Here's how the part is built. I have some questions about the finished solid (model axes, mm). A direction names the side the tool comes from. Give positions to 0.01 mm unless a question says otherwise; leave off trailing zeros. Loops run counter-clockwise (first coordinate to the right, second up) from the corner with the lowest first, then second, coordinate; pieces in that order, holes last.
Q1. Thinking about a two-plate mould opening in Z: for faces 1 (the face through (-68, 52, 0)), 2 (the face through (-67.56, 32.18, 8.35)), 3 (the face through (-68, 52, 44)), 4 (the face through (-75, 54.741, 22)), which applies, pulls with the +Z half, pulls with the -Z half, needs draft (parallel to the pull), parting line crosses it, or undercut?
Q2. Suppose I cut it at A-A (z = 8). List the corners of the cut face in (x, y) for me, and give its area (3 significant figures).
Q3. Suppose I cut it at C-C (z = 18). List the corners of the cut face in (x, y) for me.
Q4. Suppose I cut it at B-B (y = 56). List the corners of the cut face in (x, z) for me.
Q5. Suppose I cut it at D-D (x = -77.5). List the corners of the cut face in (y, z) for me.
Q6. I'm going to push flat-ended pins straight in: P1, Ø3.5, axis at x = -73.09, z = 15.57, coming from the +Y side; P2, Ø5, axis at x = -73.09, z = 27.57, coming from the -Y side; P3, Ø3.5, axis at y = 33.74, z = 40, coming from the -X side. Where does each tip first touch, or does it pass through?
Q7. I need wall thicknesses on probe 1 along Y at (x, z) = (-67.15, 40); probe 2 along Z at (x, y) = (-71.75, 57.5); probe 3 along Y at (x, z) = (-78.5, 36.5). Which ranges of each line are inside material? Lowest first, please.
Q8. For faces 5 (the face through (-67.6, 32.3, 39.3)), 6 (the face through (-69.585, 41, 22)), which set-ups out of +Z, -Z, +X, -X, +Y, -Y let a thin tool reach every point of the face, with its end or its side?
```python
from build123d import *

# Parameters (mm, degrees)
BOSS_EXTRUDE1_DEPTH = 44
SKETCH3_R           = 1.6
CUT_EXTRUDE2_DEPTH  = 10
SKETCH2_R           = 1.6
CUT_EXTRUDE3_DEPTH  = 10


with BuildPart() as part:
    # Sketch1 → Boss-Extrude1 (new body)
    with BuildSketch(Plane.XY):
        Polygon((-80.585156419, 60.740798274), (-80.585156419, 54.740798274), (-69.585156419, 54.740798274), (-69.585156419, 26.740798274), (-65.585156419, 26.740798274), (-65.585156419, 60.740798274), align=None)
    extrude(amount=BOSS_EXTRUDE1_DEPTH)

    # Sketch3 → Cut-Extrude2 (cut)
    with BuildSketch(Plane(origin=(-65.585156419, 0, 0), x_dir=(0, 0, -1), z_dir=(1, 0, 0))):
        with Locations((-40, 33.740798274)):
            Circle(SKETCH3_R)
        with Locations((-8, 33.740798274)):
            Circle(SKETCH3_R)
    extrude(amount=-CUT_EXTRUDE2_DEPTH, mode=Mode.SUBTRACT)

    # Sketch2 → Cut-Extrude3 (cut)
    with BuildSketch(Plane(origin=(0, 60.740798274, 0), x_dir=(1, 0, 0), z_dir=(0, 1, 0))):
        with Locations(Location((-73.085156419, -3.571673595, 0), (0, 0, 180))):
            Circle(SKETCH2_R)
        with Locations(Location((-73.085156419, -15.571673595, 0), (0, 0, 180))):
            Circle(SKETCH2_R)
        with Locations(Location((-73.085156419, -27.571673595, 0), (0, 0, 180))):
            Circle(SKETCH2_R)
        with Locations(Location((-73.085156419, -39.571673595, 0), (0, 0, 180))):
            Circle(SKETCH2_R)
    extrude(amount=-CUT_EXTRUDE3_DEPTH, mode=Mode.SUBTRACT)


solid = part.part
```
Solutions:
1. face 1: pulls with the -Z half
1. face 2: undercut
1. face 3: pulls with the +Z half
1. face 4: needs draft
2. outline: (-80.59, 54.74) - (-69.59, 54.74) - (-69.59, 35.34) - (-65.59, 35.34) - (-65.59, 60.74) - (-80.59, 60.74) - close; (-69.59, 26.74) - (-65.59, 26.74) - (-65.59, 32.14) - (-69.59, 32.14) - close
2. area: 189 mm2
3. outline: (-80.59, 54.74) - (-69.59, 54.74) - (-69.59, 26.74) - (-65.59, 26.74) - (-65.59, 60.74) - (-80.59, 60.74) - close
4. outline: (-80.59, 0) - (-65.59, 0) - (-65.59, 44) - (-80.59, 44) - close; hole circle Ø3.2 at (-73.09, 3.57); hole circle Ø3.2 at (-73.09, 15.57); hole circle Ø3.2 at (-73.09, 27.57); hole circle Ø3.2 at (-73.09, 39.57)
5. outline: (54.74, 0) - (60.74, 0) - (60.74, 44) - (54.74, 44) - close
6. P1: stops at y = 60.74
6. P2: stops at y = 54.74
6. P3: stops at x = -69.59
7. probe 1: y = 26.74 to 32.14, 35.34 to 60.74
7. probe 2: z = 0 to 2.69, 4.45 to 14.69, 16.45 to 26.69, 28.45 to 38.69, 40.45 to 44
7. probe 3: y = 54.74 to 60.74
8. face 5: +X, -X
8. face 6: +Z, -Z, -X, -Y
